Answer from the drawing. Dimensions are ordinates in mm from the lowest x, y and z of the part. A direction names the side the tool comes from. Round coordinates to 2 decimals unless told otherwise and drop trailing zeros. Loops run counter-clockwise (first coordinate to the right, second up) from the corner with the lowest first, then second, coordinate; pieces in that order, holes last. Notation, with made-up numbers: M -14.5,52 L 40.5,52 A19 ccw 40.5,72 Z; hole C 43,84.5 d8. An arc over 180 degrees is marked long. Answer as a JSON object with one key per item and string values.
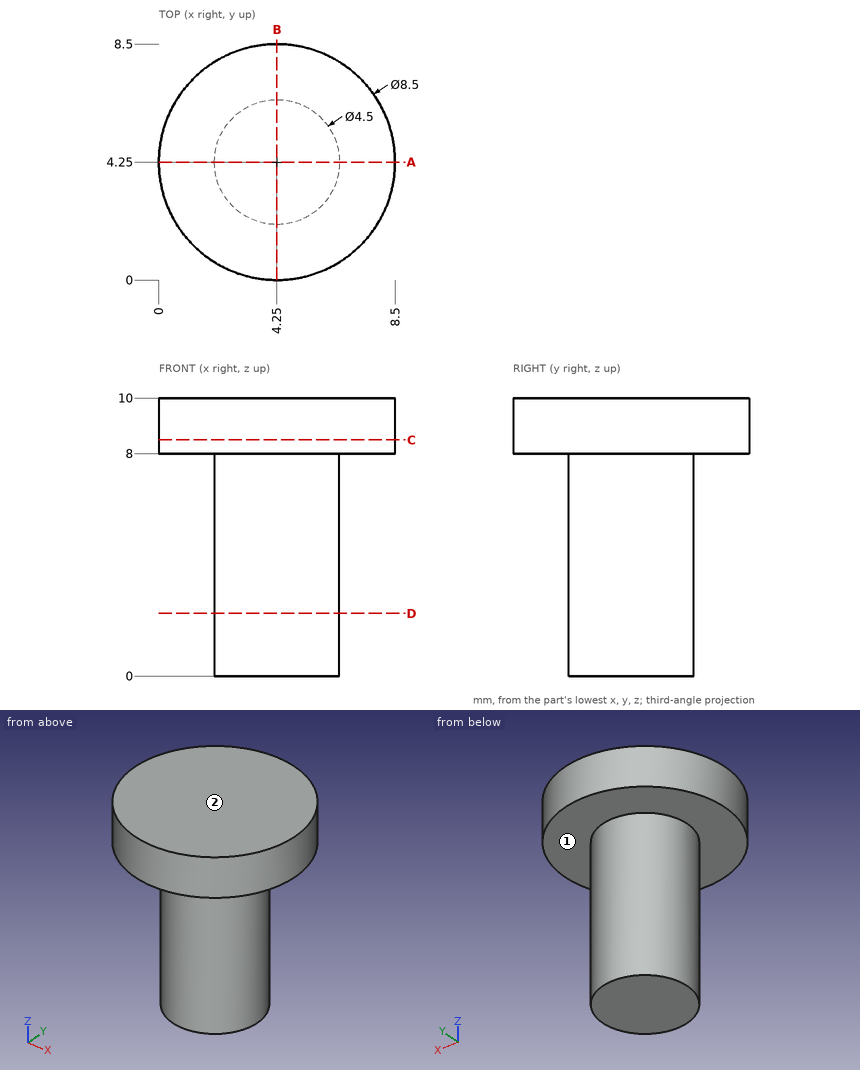
Item 1: The part is cut by section A-A (y = 4.25). Give the vertices of the cut face in (x, z).
Values follow:
{"outline": "M 0,8 L 2,8 L 2,0 L 6.5,0 L 6.5,8 L 8.5,8 L 8.5,10 L 0,10 Z"}
Item 2: Straight lines are drawn through the part: line 1 (Z direction, x = 3.75, y = 1.75); line 2 (X direction, y = 6, z = 3.5). For each, find the intervals that lie inside material, in ascending order.
Values follow:
{"line 1": "8 to 10", "line 2": "2.84 to 5.66"}
Item 3: The part is cut by section D-D (z = 2.25). Give the vertices of the cut face in (x, y).
Values follow:
{"outline": "C 4.25,4.25 d4.5"}
Item 4: Flat-ended cylindrical pins translate along their axes: P1, Ø3, axis at y = 1.5, z = 4, coming from the +X side; P2, Ø4, axis at x = 2, z = 5.5, coming from the -Y side; P3, Ø1.5, axis at y = 6, z = 5.5, coming from the +X side; P4, Ø4, axis at x = 6, y = 6, coming from the -Z side. Find the tip coordinate at first contact, or state that the pin passes through.
Values follow:
{"P1": "x = 6.12", "P2": "y = 2.01", "P3": "x = 6.27", "P4": "z = 0"}
Item 5: Which of the six approach directions +Z, -Z, +X, -X, +Y, -Y give full straight-line access (tool end or side, diameter ignored) to the marked faces 1 and 2?
Values follow:
{"face 1": "-Z", "face 2": "+Z, +X, -X, +Y, -Y"}
Item 6: The part is cut by section C-C (z = 8.5). Give the vertices of the cut face in (x, y).
Values follow:
{"outline": "C 4.25,4.25 d8.5"}
